Can you work these out from the model? Positions are in its coordinate system, mm. A direction names the side the tool comes from. Give positions to 0.01 mm unless a question says otherwise; leave off trailing zeros. Write each loop counter-clockwise with the first axis right and the second up, starting at its lowest first coordinate (ties: lowest second). Pieces come first, ordered by that corner, then holes. Notation, with made-up numbers: (-23.75, 70) -> (4.25, 70) arc R16 cw to (4.25, 76) -> close; hole circle Ø4 at (45.5, 88). An arc over 180 degrees is marked (long way). Answer as CSV lines item,"result". Start each with the question number.
1. If we mould it in two halves opening along X, with no side actions, what happens to faces 1 (the face through (-6.35, 2, 15)), 2 (the face through (-0.38, 2.474, 19.173)), 3 (the face through (-0.38, 2.47, -15.75)), 4 (the face through (0, 2, -22.225))? For each: pulls with the +X half, pulls with the -X half, needs draft (parallel to the pull), parting line crosses it, or undercut.
2. I'm going to push flat-ended pins straight in: P1, Ø1, axis at y = 2.5, z = -5, coming from the -X side; P2, Ø2, axis at x = 0, z = -17.46, coming from the -Y side. Where does each tip first touch, or does it pass through?
3. If we section it at D-D on x = -4.25: Write out the boundary of the cut face in (y, z) (3 decimals), plus the area to 3 significant figures.
4. On a 3-axis mill with a long thin cutter (end or side, diameter ignored), from which of +Z, -Z, +X, -X, +Y, -Y can I reach the whole of each face in a straight line? I mean faces 5 (the face through (-3.471, 1.735, -0.178)), 6 (the face through (6.35, 2, 0)). Say none if no direction works.
5. If we section it at B-B on y = 1.1: Count the separate pieces of the cut face and the enclosed holes in it, plus the area to 3 significant figures.
6. I need wall thicknesses on line 1 (Z direction, x = 0, y = 2.6) (3 decimals); line 2 (Z direction, x = -6, y = 0.3) (3 decimals); line 3 (Z direction, x = -0.5, y = 1.5) (3 decimals). Which ranges of each line are inside material? Lowest first, please. Write a range as [from, to].
7. If we section it at A-A on x = 0: Write out the boundary of the cut face in (y, z) (3 decimals).
Autodesk Inventor part; units mm, degrees
ref_plane "YZ Plane" through (0, 0, 0) normal (1, 0, 0) x (0, 1, 0)
ref_plane "XZ Plane" through (0, 0, 0) normal (0, 1, 0) x (-1, 0, 0)
ref_plane "XY Plane" through (0, 0, 0) normal (0, 0, 1) x (1, 0, 0)
sketch "Sketch1" plane through (0, 0, 0) normal (0, 1, 0) x (-1, 0, 0)
  line L0 (-6.35, 22.225) -> (6.35, 22.225)
  line L1 (6.35, 22.225) -> (6.35, -22.225)
  line L2 (6.35, -22.225) -> (-6.35, -22.225)
  line L3 (-6.35, -22.225) -> (-6.35, 22.225)
  line L4 (-6.35, 22.225) -> (6.35, -22.225) construction
  line L5 (6.35, 22.225) -> (-6.35, -22.225) construction
  line L6 (-4.7625, 9.525) -> (4.7625, 9.525) construction
  line L7 (4.7625, 9.525) -> (4.7625, -9.525) construction
  line L8 (4.7625, -9.525) -> (-4.7625, -9.525) construction
  line L9 (-4.7625, -9.525) -> (-4.7625, 9.525) construction
  line L10 (-4.7625, 9.525) -> (4.7625, -9.525) construction
  line L11 (4.7625, 9.525) -> (-4.7625, -9.525) construction
  point P0 (0, 0)
  dimension "d0" = 12.7
  dimension "d1" = 44.45
  dimension "d2" = 9.525
  dimension "d3" = 19.05
extrude "Extrusion1" add sketch "Sketch1" along normal blind 3.175
chamfer "Chamfer1" distance 3.175 distance2 6.35 1 edges at (-6.35, 0, 0) measured on face at (-6.35, 1.0583, -7.4083)
fillet "Fillet1" radius 3.175 1 edges at (-0.0005, 0, 0)
sketch "Sketch2" plane through (0, 3.175, 0) normal (0, 1, 0) x (1, 0, 0)
  line L0 (0, -17.4625) -> (0, -17.4625) construction
  line L1 (0, -17.4625) -> (0, 17.4625) construction
  line L2 (0, 17.4625) -> (0, 17.4625) construction
  line L3 (0, 17.4625) -> (0, -17.4625) construction
  line L4 (0, -17.4625) -> (0, 17.4625) construction
  line L5 (0, -17.4625) -> (0, 17.4625) construction
  circle A0 centre (0, -17.4625) radius 1.7526
  circle A1 centre (0, 17.4625) radius 1.7526
  circle A2 centre (0, -17.4625) radius 1.7526
  circle A3 centre (0, 17.4625) radius 1.7526
  line L6 (6.35, 12.7) -> (-6.35, 12.7)
  line L7 (-6.35, 12.7) -> (-6.35, 22.225)
  line L8 (-6.35, 22.225) -> (6.35, 22.225)
  line L9 (6.35, 22.225) -> (6.35, 12.7)
  line L10 (6.35, 12.7) -> (-6.35, 22.225) construction
  line L11 (-6.35, 12.7) -> (6.35, 22.225) construction
  line L12 (-6.35, 22.225) -> (-6.35, -22.225)
  line L13 (-6.35, 0) -> (6.35, 0) construction
  line L14 (6.35, -22.225) -> (6.35, 22.225)
  line L15 (6.35, -12.7) -> (-6.35, -12.7)
  line L16 (-6.35, -12.7) -> (-6.35, -22.225)
  line L17 (-6.35, -22.225) -> (6.35, -22.225)
  line L18 (6.35, -22.225) -> (6.35, -12.7)
  line L19 (6.35, -12.7) -> (-6.35, -22.225) construction
  line L20 (-6.35, -12.7) -> (6.35, -22.225) construction
  point P0 (0, 0)
  point P1 (0, 17.4625)
  point P2 (0, -17.4625)
  point P3 (0, -17.4625)
  point P4 (0, -17.4625)
  point P5 (6.35, -12.7)
  point P6 (-6.35, -12.7)
  point P7 (-6.35, -22.225)
  dimension "d10" = 0
  dimension "d11" = 34.925
  dimension "d12" = 3.5052
  dimension "d15" = 34.925
  dimension "d18" = 0
  dimension "d21" = 12.7
  dimension "d22" = 9.525
extrude "Extrusion2" add sketch "Sketch2" against normal up to surface (3.175 mm away) contours A0 | A1 | L6 L7 L8 L9 | L14 L17 L12 L15
extrude "Extrusion3" cut sketch "Sketch2" against normal through all contours A0 | A1
chamfer "Chamfer2" distance 1.524 angle 49 2 edges at (-1.7526, 0, 17.4625) (-1.7526, 0, -17.4625) measured on face at (4.483, 0, 4.2333)
equation "\"d15\" = d11"
properties part number "ramp" material "UHMW, White"
Computed values:
1,face 1,"pulls with the -X half"
1,face 2,"undercut"
1,face 3,"undercut"
1,face 4,"needs draft"
2,P1,"stops at x = -6"
2,P2,"passes through"
3,outline,"(0, -22.225) -> (3.175, -22.225) -> (3.175, 22.225) -> (0, 22.225) -> (0, 12.7) -> (2.125, 12.7) -> (2.125, -12.7) -> (0, -12.7) -> close"
3,area,"87.2 mm2"
4,face 5,"-X, -Y"
4,face 6,"+Z, -Z, +X, +Y, -Y"
5,separate pieces,"1"
5,enclosed holes,"2"
5,area,"425 mm2"
6,line 1,"z = [-22.225, -19.215], [-15.71, 15.71], [19.215, 22.225]"
6,line 2,"z = [-22.225, -12.7], [12.7, 22.225]"
6,line 3,"z = [-22.225, -19.371], [-15.554, 15.554], [19.371, 22.225]"
7,outline,"(0, -22.225) -> (3.175, -22.225) -> (3.175, -19.215) -> (1.753, -19.215) -> (0, -20.739) -> close; (0, -14.186) -> (1.753, -15.71) -> (3.175, -15.71) -> (3.175, 15.71) -> (1.753, 15.71) -> (0, 14.186) -> (0, 12.7) -> (0.09, 12.7) -> (0.09, -12.7) -> (0, -12.7) -> close; (0, 20.739) -> (1.753, 19.215) -> (3.175, 19.215) -> (3.175, 22.225) -> (0, 22.225) -> close"
